Design review of the part built by this model. Coordinates are the model's own, in mm. Face numbers are marked on the shaded views. A direction names the side the tool comes from. Coordinates: 2 decimals unless noted, no trailing zeros. Write each loop counter-clockwise with the first axis right and the second up, starting at its lowest first coordinate (ties: lowest second). Pieces come first, ordered by that corner, then holes.
Q1. The part is to be moulded in two halves that separate along X. For the marked faces 5, 6, 7 and 8, say which applies: +X half, -X half, draft (parallel to the pull), parting line (faces both ways), or undercut.
Q2. Clearance check with flat-ended pins moving along their axes: pin 1 Ø2 at (y, z) = (15, 33.5) entering from -X; pin 2 Ø10 at (x, y) = (-9.5, 18.5) entering from -Z; pin 3 Ø4 at (y, z) = (14, -28) entering from -X. State where each tip first meets the part, or that it passes through.
Q3. Add section B-B, the plane z = 7.5. Give the boundary of the cut face in (x, y), plus the area to 3 significant figures.
Q4. Machinability: for the marked faces 1, 2, 3 and 4, which of the approach directions +Z, -Z, +X, -X, +Y, -Y give a long, thin tool a straight path to every point of the face, cutting with its end or side? Answer none if there is none.
Q5. Add section A-A, the plane z = -34.5. Give the boundary of the cut face in (x, y), plus the area to 3 significant figures.
Q6. Add section C-C, the plane x = 21.5. Give the boundary of the cut face in (y, z).
Q7. To check wall thickness, follow probe 1 along X at (y, z) = (9.5, 0); probe 2 along X at (y, z) = (11.25, -42.5); probe 3 along Z at (x, y) = (6, 16). State the ranges of each line that lie inside material, in increasing order.
from build123d import *

# Parameters (mm, degrees)
SKETCH_16_W              = 20
SKETCH_16_H              = 30
EXTRUDE_2_DEPTH          = 30
PATTERN_CIRCULAR_3_COUNT = 15


with BuildPart() as part:
    # 草图16 → 旋转5 (revolve)
    with BuildSketch(Plane.XY, mode=Mode.PRIVATE) as revolve_5_sk:
        with Locations((-30.151216768, 15)):
            Rectangle(SKETCH_16_W, SKETCH_16_H)
    revolve(revolve_5_sk.sketch.rotate(Axis((-0.151216768, 0, 0), (0, 1, 0)), 270), axis=Axis((-0.151216768, 0, 0), (0, 1, 0)))

    # 草图17 → 凸台-拉伸2 (add, through all)
    with BuildSketch(Plane(origin=(0, 30, 0), x_dir=(1, 0, 0), z_dir=(0, 1, 0))):
        with BuildLine():
            Line((-48.6676208, -0.245209253), (-39.833774171, -5.029377496))
            ThreePointArc((-39.833774171, -5.029377496), (-40.151130439, 0.083104397), (-39.81253347, 5.194223472))
            Line((-39.81253347, 5.194223472), (-48.6676208, -0.245209253))
        make_face()
    extrude_2 = extrude(amount=-EXTRUDE_2_DEPTH)

    # 阵列(圆周)3: 凸台-拉伸2 ×15 about axis
    pattern_circular_3_axis = Axis((-0.151216768, 0, 0), (0, 1, 0))
    for i in range(1, PATTERN_CIRCULAR_3_COUNT):
        add(extrude_2.rotate(pattern_circular_3_axis, i * 360 / PATTERN_CIRCULAR_3_COUNT))


solid = part.part
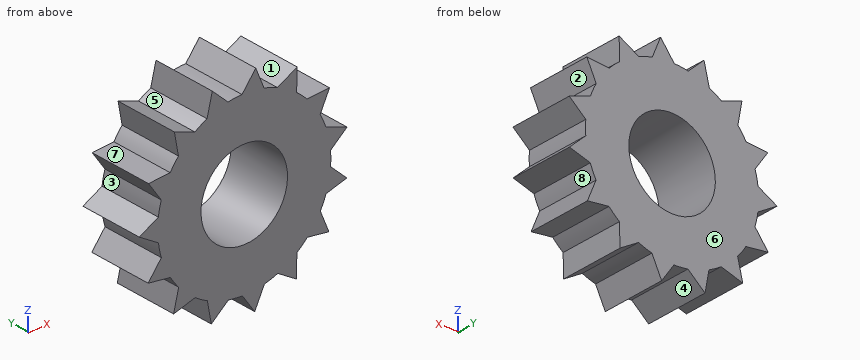
Here are the results:
1. face 5: undercut
1. face 6: draft
1. face 7: -X half
1. face 8: +X half
2. pin 1: stops at x = -32.12
2. pin 2: stops at z = -45.32
2. pin 3: stops at x = -31.38
3. outline: (-39.44, 0) - (-18.69, 0) - (-18.69, 30) - (-39.44, 30) - close; (18.39, 0) - (44.6, 0) - (44.6, 30) - (18.39, 30) - close
3. area: 1,410 mm2
4. face 1: +Z, +Y, -Y
4. face 2: +X, +Y, -Y
4. face 3: -X, +Y, -Y
4. face 4: -Z, +Y, -Y
5. outline: (-32.46, 0) - (-28.08, 0) - (-28.08, 30) - (-32.46, 30) - close; (-20.39, 0) - (24.1, 0) - (24.1, 30) - (-20.39, 30) - close
5. area: 1,470 mm2
6. outline: (0, -40.67) - (30, -40.67) - (30, 40.37) - (0, 40.37) - close
7. probe 1: x = -48.27 to -20.15, 19.85 to 39.85
7. probe 2: x = -16.03 to -11.19, 0.72 to 7.44
7. probe 3: z = -45.51 to -19.03, 19.03 to 46.2
